from build123d import *

# Parameters (mm, degrees)
SKETCH_R        = 1.6
PAD_DEPTH       = 3
POCKET014_DEPTH = 3.001
CHAMFER059_SIZE = 1
CHAMFER_SIZE    = 1


with BuildPart() as part:
    # Sketch → Pad (new body)
    with BuildSketch(Plane.YZ.offset(40)):
        with BuildLine():
            Line((8, 320), (31, 320))
            Line((31, 320), (31, 315))
            ThreePointArc((31, 315), (33.343146, 309.343146), (39, 307))
            Line((75, 307), (39, 307))
            Line((75, 140), (75, 307))
            Line((-5, 140), (75, 140))
            Line((-5, 156), (-5, 140))
            Line((-5, 156), (0, 156))
            ThreePointArc((0, 156), (4, 160), (0, 164))
            Line((0, 164), (-5, 164))
            Line((-5, 180), (-5, 164))
            Line((8, 180), (-5, 180))
            Line((8, 320), (8, 180))
        make_face()
        with Locations((19.5, 315)):
            Circle(SKETCH_R, mode=Mode.SUBTRACT)
        with Locations((70, 292)):
            Circle(SKETCH_R, mode=Mode.SUBTRACT)
        with Locations((70, 155)):
            Circle(SKETCH_R, mode=Mode.SUBTRACT)
    extrude(amount=PAD_DEPTH)

    # Sketch158 (on Face18 of Pad) → Pocket014 (cut, through all)
    with BuildSketch(Plane.YZ.offset(43)):
        with BuildLine():
            ThreePointArc((54, 140), (56.5, 137.5), (59, 140))
            Line((59, 140), (59, 160))
            ThreePointArc((59, 160), (56.5, 162.5), (54, 160))
            Line((54, 160), (54, 140))
        make_face()
    extrude(amount=-POCKET014_DEPTH, mode=Mode.SUBTRACT)

    # Chamfer059
    chamfer059_edges = [part.edges().sort_by_distance(p)[0] for p in [
        (41.5, 54, 140),
        (41.5, 59, 140),
    ]]
    chamfer(chamfer059_edges, length=CHAMFER059_SIZE)

    # Chamfer
    chamfer_edges = [part.edges().sort_by_distance(p)[0] for p in [
        (41.5, -5, 180),
        (41.5, 8, 180),
        (41.5, -5, 140),
        (41.5, -5, 156),
        (41.5, 75, 140),
        (41.5, 75, 307),
        (41.5, 31, 320),
        (41.5, 8, 320),
    ]]
    chamfer(chamfer_edges, length=CHAMFER_SIZE)


solid = part.part
Verification items for the finished model (mm, model axes). A direction names the side the tool comes from. Give positions to 0.01 mm unless a question says otherwise; leave off trailing zeros. Order: outer loops, then holes, each group sorted by start corner. A loop starts at its lowest first (then second) coordinate and runs counter-clockwise, first axis right, second up. Notation, with made-up numbers: M -37,34.5 L 15,34.5 A16 ccw 15,60.5 Z; hole C 46.25,53 d2. An arc over 180 degrees is marked long. Answer as a JSON object with one key per item and string values. Group by question number.
1) Depth check by flat-ended pin: pin 1 Ø1.5 at (x, y) = (42, 2.5) entering from +Z; pin 2 Ø1.5 at (x, z) = (41, 271) entering from -Y; pin 3 Ø4 at (y, z) = (70, 155) entering from -X. Enter the tip coordinate at first touch or a pass-through.
2) Cross-section at D-D (z = 266). Enter the section's corners in (x, y), then the cut area to 3 significant figures.
3) Scan lines: line 1 along Z through (x, y) = (41.95, 70); line 2 along Y through (x, z) = (42.05, 155); line 3 along Z through (x, y) = (41.55, 19.5). Record each from-to range of solid material in increasing order. Write a range as [from, to].
4) Cross-section at A-A (y = 70). Enter the section's corners in (x, z), then the cut area to 3 significant figures.
5) Access from +Z, -Z, +X, -X, +Y, -Y to the whole of each face (thin tool, end or side, straight path). Record for faces 1 (the face through (41, 57, 307)), 2 (the face through (42, 59, 150)), 3 (the face through (41, -2, 164)).
6) Cross-section at B-B (x = 41). Give the number of separate pieces and of enclosed holes in the cut face, then the cut area to 3 significant figures.
7) Cross-section at C-C (y = 19.5). Enter the section's corners in (x, z), then the cut area to 3 significant figures.
Result sheet:
{
 "1": {"pin 1": "stops at z = 180", "pin 2": "stops at y = 8", "pin 3": "stops at x = 40"},
 "2": {"outline": "M 40,8 L 43,8 L 43,75 L 40,75 Z", "area": "201 mm2"},
 "3": {"line 1": "z = [140, 153.4], [156.6, 290.4], [293.6, 307]", "line 2": "y = [-5, 54], [59, 68.4], [71.6, 75]", "line 3": "z = [140, 313.4], [316.6, 320]"},
 "4": {"outline": "M 40,140 L 43,140 L 43,153.4 L 40,153.4 Z; M 40,156.6 L 43,156.6 L 43,290.4 L 40,290.4 Z; M 40,293.6 L 43,293.6 L 43,307 L 40,307 Z", "area": "482 mm2"},
 "5": {"face 1": "+Z, +X, -X, +Y", "face 2": "-Z, +X, -X", "face 3": "+X, -X, -Y"},
 "6": {"separate pieces": "1", "enclosed holes": "3", "area": "11,800 mm2"},
 "7": {"outline": "M 40,140 L 43,140 L 43,313.4 L 40,313.4 Z; M 40,316.6 L 43,316.6 L 43,320 L 40,320 Z", "area": "530 mm2"}
}
